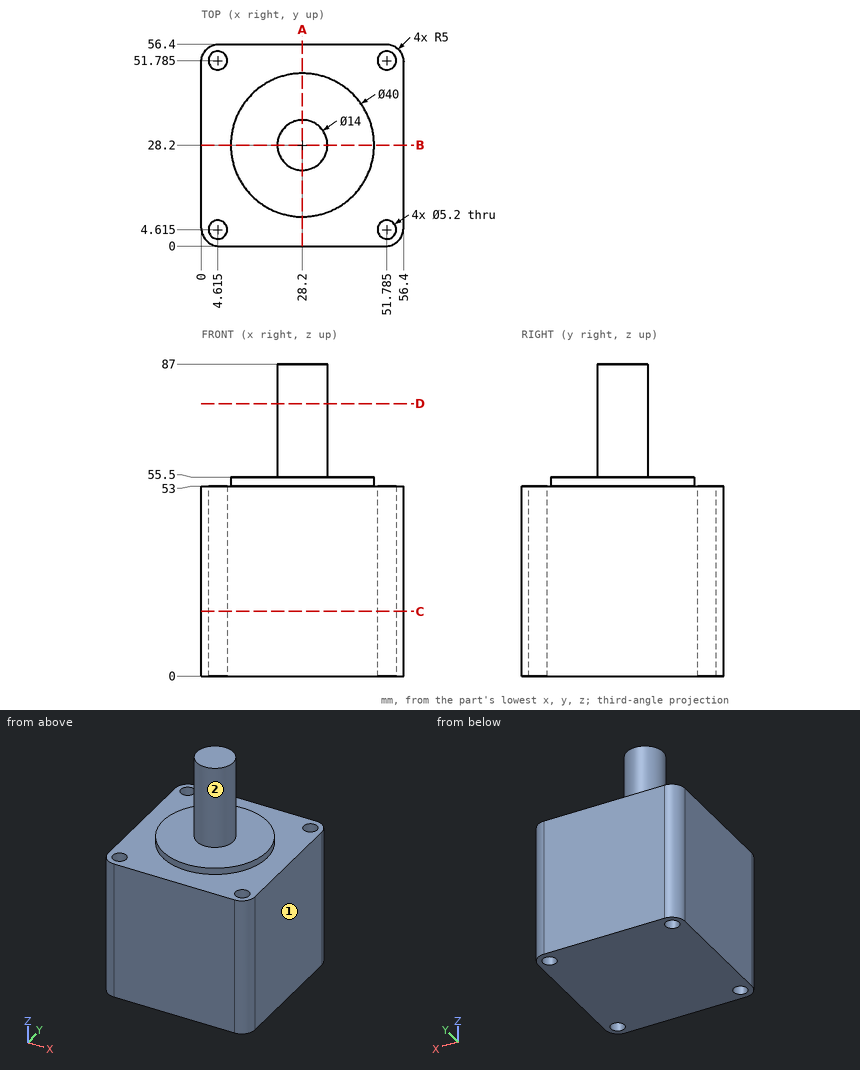
Source: three-view drawing plus pictorial views. Frame: mm from the lowest corner of the part. A direction names the side the tool comes from. Round coordinates to 2 decimals unless told otherwise and drop trailing zeros. Write each loop counter-clockwise with the first axis right and the second up, starting at its lowest first coordinate (ties: lowest second). Pieces come first, ordered by that corner, then holes. Notation, with made-up numbers: M -17,51 L 12,51 A27 cw 12,90 Z; hole C 31.5,12 d4. An arc over 180 degrees is marked long. Use CSV: the item, a comma, the result in double quotes. Start each with the question number.
Q1. Cut plane C-C on z = 18. Output: boundary loops of the cut face in (x, y) (3 decimals).
Q2. Access query for the marked faces 1 and 2. Directions: +Z, -Z, +X, -X, +Y, -Y. A direction counts if a zero-diameter tool reaches every point of the face in a straight line with its end or side. Return the directions, or none.
Q3. Cut plane D-D on z = 76. Output: boundary loops of the cut face in (x, y).
Q4. Line query: line 1 (X direction, y = 5.5, z = 40.5); line 2 (Z direction, x = 14, y = 8.5); line 3 (Z direction, x = 9, y = 28). Output: solid intervals per line, ascending. Write a range as from..to.
Q5. First-contact query: P1, Ø7, axis at x = 51.785, y = 51.785, coming from the +Z side; P2, Ø8, axis at x = 45, y = 39, coming from the +Z side; P3, Ø3, axis at x = 51.785, y = 4.615, coming from the -Z side. Flat tips, straight axial feed; report the tip coordinate or a pass-through.
Q6. Cut plane A-A on x = 28.2. Output: boundary loops of the cut face in (y, z).
Results found:
1,outline,"M 0,5 A5 ccw 5,0 L 51.4,0 A5 ccw 56.4,5 L 56.4,51.4 A5 ccw 51.4,56.4 L 5,56.4 A5 ccw 0,51.4 Z; hole C 4.615,4.615 d5.2; hole C 4.615,51.785 d5.2; hole C 51.785,4.615 d5.2; hole C 51.785,51.785 d5.2"
2,face 1,"+Z, -Z, +X, +Y, -Y"
2,face 2,"+Z"
3,outline,"C 28.2,28.2 d14"
4,line 1,"0..2.17, 7.06..49.34, 54.23..56.4"
4,line 2,"0..53"
4,line 3,"0..55.5"
5,P1,"z = 53"
5,P2,"z = 55.5"
5,P3,"through"
6,outline,"M 0,0 L 56.4,0 L 56.4,53 L 48.2,53 L 48.2,55.5 L 35.2,55.5 L 35.2,87 L 21.2,87 L 21.2,55.5 L 8.2,55.5 L 8.2,53 L 0,53 Z"
